Verification items for the finished model (mm, model axes). A direction names the side the tool comes from. Coordinates: 2 decimals unless noted, no trailing zeros. Order: outer loops, then holes, each group sorted by start corner. A loop starts at its lowest first (then second) coordinate and runs counter-clockwise, first axis right, second up. Notation, with made-up numbers: M 46.25,88 L 69.25,88 A10 ccw 69.25,96 Z; hole C 58.25,80.5 d9. An arc over 180 degrees is marked long. Answer as a JSON object with one key per item and string values. Group by question number.
(1) Cross-section at C-C (x = 145.5). Enter the section's corners in (y, z).
(2) Cross-section at A-A (y = 0.8). Enter the section's corners in (x, z), plus the area to 3 significant figures.
(3) Material ranges on line 1 (X direction, y = 1.2, z = -65); line 2 (X direction, y = 0.9, z = 0); line 3 (Z direction, x = 60, y = 1.25), recorded low to high.
(4) Cross-section at B-B (z = -4). Enter the section's corners in (x, y).
(5) Access from +Z, -Z, +X, -X, +Y, -Y to the whole of each face (thin tool, end or side, straight path). Record for faces 1 (the face through (114.66, 1.01, 1.87)), 2 (the face through (0.45, 0.99, 1.43)).
(6) Mould release check, pull along X, two halves, no side actions. Record for faces 3 (the face through (107.45, 0.99, -4.29)), 4 (the face through (77, 2, -34)), 5 (the face through (140.99, 0.99, -34.58)): released by +X, released by -X, zero draft, split by the parting line, or undercut.
(7) Cross-section at D-D (z = -55). Enter the section's corners in (x, y), plus the area to 3 significant figures.
(8) Gauge pin test, flat ends, axial feed: pin 1 Ø1.8 at (x, z) = (0, 0) entering from -Y; pin 2 Ø1 at (x, y) = (117, 1) entering from +Z; pin 3 Ø1 at (y, z) = (1, -5) entering from +X; pin 4 Ø1 at (x, y) = (70, 1) entering from +Z. Record the tip position at first contact, or that the pin passes through.
from build123d import *

# Parameters (mm, degrees)
SKETCH_1_R      = 1.5
EXTRUDE_1_DEPTH = 2
FILLET_1_R      = 10
FILLET_2_R      = 10
FILLET_3_R      = 10
FILLET_4_R      = 10


with BuildPart() as part:
    # 草图1 → 凸台-拉伸1 (new body)
    with BuildSketch(Plane(origin=(0, 0, 0), x_dir=(1, 0, 0), z_dir=(0, 1, 0))):
        with BuildLine():
            Line((-2.439592735, 1.034836841), (25.627407265, 67.201836841))
            ThreePointArc((25.627407265, 67.201836841), (26.60409495, 68.376617346), (28.067, 68.817))
            Line((28.067, 68.817), (124.714, 68.817))
            ThreePointArc((124.714, 68.817), (126.17690505, 68.376617346), (127.153592735, 67.201836841))
            Line((127.153592735, 67.201836841), (155.220592735, 1.034836841))
            ThreePointArc((155.220592735, 1.034836841), (154.990617346, -1.46290505), (152.781, -2.65))
            Line((152.781, -2.65), (114.3905, -2.65))
            Line((114.3905, -2.65), (100.3905, 11.35))
            Line((100.3905, 11.35), (52.3905, 11.35))
            Line((52.3905, 11.35), (38.3905, -2.65))
            Line((38.3905, -2.65), (0, -2.65))
            ThreePointArc((0, -2.65), (-2.209617346, -1.46290505), (-2.439592735, 1.034836841))
        make_face()
        with Locations(Location((0, 0, 0), (0, 0, 270))):
            Circle(SKETCH_1_R, mode=Mode.SUBTRACT)
        with Locations(Location((152.781, 0, 0), (0, 0, 270))):
            Circle(SKETCH_1_R, mode=Mode.SUBTRACT)
        with Locations(Location((28.067, 66.167, 0), (0, 0, 270))):
            Circle(SKETCH_1_R, mode=Mode.SUBTRACT)
        with Locations(Location((124.714, 66.167, 0), (0, 0, 90))):
            Circle(SKETCH_1_R, mode=Mode.SUBTRACT)
    extrude(amount=EXTRUDE_1_DEPTH)

    # 圆角1
    fillet_1_edges = [part.edges().sort_by_distance(p)[0] for p in [
        (38.3905, 1, 2.65),
    ]]
    fillet(fillet_1_edges, radius=FILLET_1_R)

    # 圆角2
    fillet_2_edges = [part.edges().sort_by_distance(p)[0] for p in [
        (52.3905, 1, -11.35),
    ]]
    fillet(fillet_2_edges, radius=FILLET_2_R)

    # 圆角3
    fillet_3_edges = [part.edges().sort_by_distance(p)[0] for p in [
        (100.3905, 1, -11.35),
    ]]
    fillet(fillet_3_edges, radius=FILLET_3_R)

    # 圆角4
    fillet_4_edges = [part.edges().sort_by_distance(p)[0] for p in [
        (114.3905, 1, 2.65),
    ]]
    fillet(fillet_4_edges, radius=FILLET_4_R)


solid = part.part
Taken from the geometry:
{
 "1": {"outline": "M 0,-23.95 L 2,-23.95 L 2,2.65 L 0,2.65 Z"},
 "2": {"outline": "M -2.44,-1.03 L 25.63,-67.2 A2.65 ccw 28.07,-68.82 L 124.71,-68.82 A2.65 ccw 127.15,-67.2 L 155.22,-1.03 A2.65 ccw 152.78,2.65 L 118.53,2.65 A10 ccw 111.46,-0.28 L 103.32,-8.42 A10 cw 96.25,-11.35 L 56.53,-11.35 A10 cw 49.46,-8.42 L 41.32,-0.28 A10 ccw 34.25,2.65 L 0,2.65 A2.65 ccw Z; hole C 0,0 d3; hole C 28.07,-66.17 d3; hole C 124.71,-66.17 d3; hole C 152.78,0 d3", "area": "8,420 mm²"},
 "3": {"line 1": "x = 24.69 to 27.12, 29.01 to 123.77, 125.66 to 128.09", "line 2": "x = -2.65 to -1.5, 1.5 to 41.03, 111.75 to 151.28, 154.28 to 155.43", "line 3": "z = -68.82 to -11.35"},
 "4": {"outline": "M -1.18,0 L 45.04,0 L 45.04,2 L -1.18,2 Z; M 107.74,0 L 153.96,0 L 153.96,2 L 107.74,2 Z"},
 "5": {"face 1": "+Z, +Y, -Y", "face 2": "+Y, -Y"},
 "6": {"face 3": "undercut", "face 4": "zero draft", "face 5": "released by +X"},
 "7": {"outline": "M 20.45,0 L 132.33,0 L 132.33,2 L 20.45,2 Z", "area": "224 mm²"},
 "8": {"pin 1": "passes through", "pin 2": "stops at z = 2.6", "pin 3": "stops at x = 153.75", "pin 4": "stops at z = -11.35"}
}
